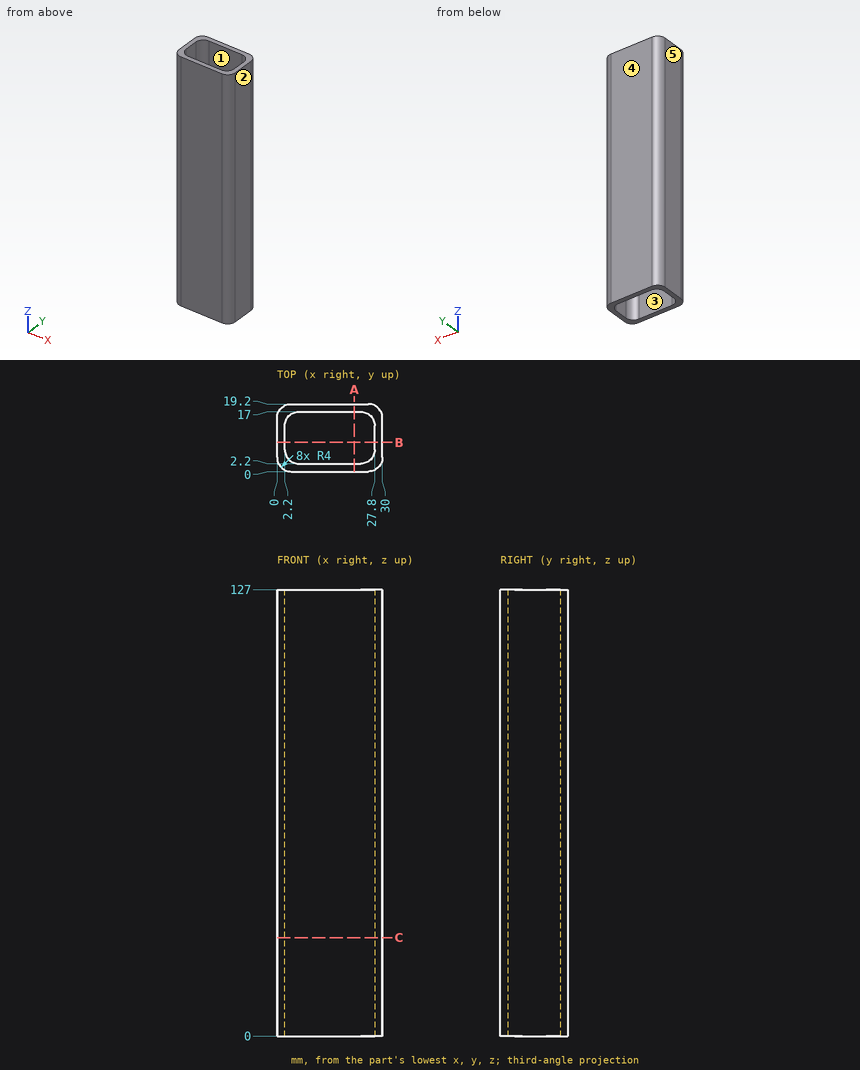
For this review, use the dimensioned drawing (mm, ordinates from the lowest corner) and the shaded views. A direction names the side the tool comes from. Coordinates: 2 decimals unless noted, no trailing zeros. Loops run counter-clockwise (first coordinate to the right, second up) from the corner with the lowest first, then second, coordinate; pieces in that order, holes last. Notation, with made-up numbers: (56, 87) - (98, 87) arc R21 ccw to (98, 114) - close; hole circle Ø3 at (59.25, 9). An arc over 180 degrees is marked (long way). Use one line per item in the form item = value. Start each with the question number.
1) Take a section at B-B (y = 8.25). State the section outline as (x, z) points.
2) For the marked faces 1 and 2, list the 3-axis set-ups (+Z, -Z, +X, -X, +Y, -Y) from which the entire face can be reached by the end or side of a thin tool; tool diameter is ignored.
3) Take a section at A-A (x = 22). State the section outline as (y, z) points.
4) For pin 1 (2 mm diameter, centred on y = 2.5, z = 38.5, fed in from +X), flat-tipped, find the tip position at first contact; note if it passes through.
5) Take a section at C-C (z = 28). State the section outline as (x, y) points, plus the area to 3 significant figures.
6) Draft analysis for pull direction Y (two halves, no side actions). For the marked faces 3, 4 and 5, state which applies: released by +Y, released by -Y, zero draft, split by the parting line, or undercut.
7) To check wall thickness, follow probe 1 along X at (y, z) = (8, 105); probe 2 along Y at (x, z) = (13, 47.5); probe 3 along Y at (x, z) = (4.25, 49.5). State the ranges of each line that lie inside material, in increasing order. Write a range as from..to.
From the geometry:
q1.outline = (0, 0) - (2.2, 0) - (2.2, 127) - (0, 127) - close; (27.8, 0) - (30, 0) - (30, 127) - (27.8, 127) - close
q2.face_1 = +Z, -Z
q2.face_2 = +Z, -Z, +X, +Y, -Y
q3.outline = (0, 0) - (2.2, 0) - (2.2, 127) - (0, 127) - close; (17, 0) - (19.2, 0) - (19.2, 127) - (17, 127) - close
q4.pin_1 = 29.97
q5.outline = (0, 4) arc R4 ccw to (4, 0) - (26, 0) arc R4 ccw to (30, 4) - (30, 15.2) arc R4 ccw to (26, 19.2) - (4, 19.2) arc R4 ccw to (0, 15.2) - close; hole (2.2, 6.2) arc R4 ccw to (6.2, 2.2) - (23.8, 2.2) arc R4 ccw to (27.8, 6.2) - (27.8, 13) arc R4 ccw to (23.8, 17) - (6.2, 17) arc R4 ccw to (2.2, 13) - close
q5.area = 197 mm2
q6.face_3 = undercut
q6.face_4 = released by +Y
q6.face_5 = zero draft
q7.probe_1 = 0..2.2, 27.8..30
q7.probe_2 = 0..2.2, 17..19.2
q7.probe_3 = 0..2.71, 16.49..19.2
